Geometry: see drawing. Coordinates: mm, zero at the bounding-box minimum. A direction names the side the tool comes from. Give positions to 0.01 mm unless a question says otherwise; leave off trailing zeros. Loops run counter-clockwise (first coordinate to the right, second up) from the corner with the lowest first, then second, coordinate; pieces in that order, holes last. Notation, with made-up numbers: (-17.75, -3) - (-8.75, -3) arc R21 ccw to (-8.75, 36) - close; hole circle Ø7 at (-19.5, 39). An arc over 180 degrees is marked (long way). Use CSV: the item, a comma, the result in double quotes. Start each with the question number.
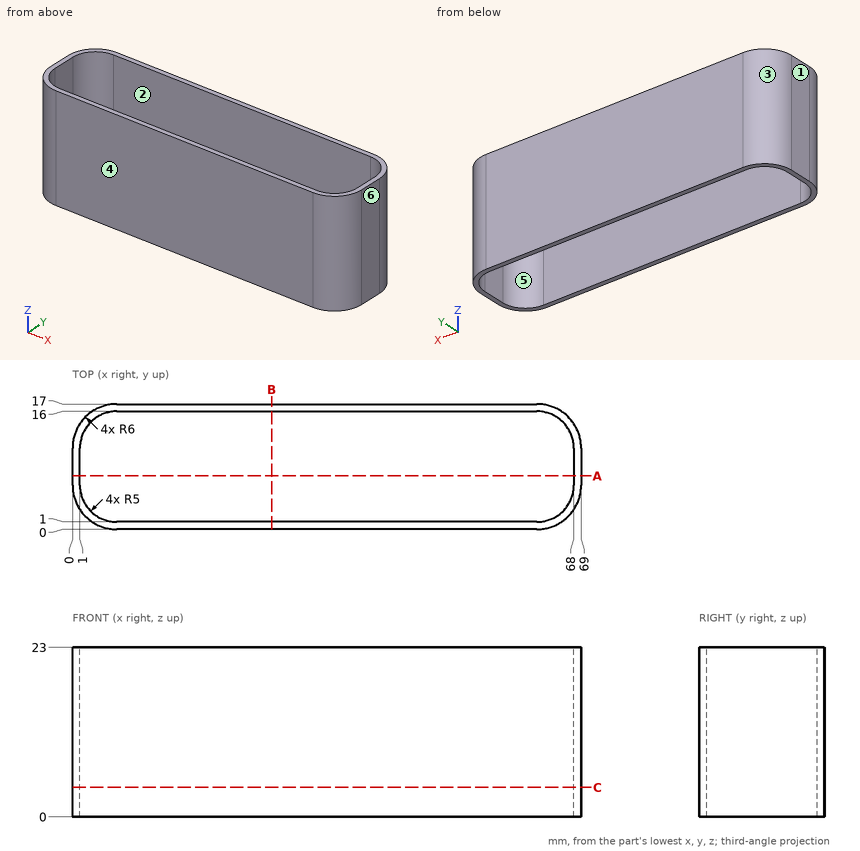
Item 1: Section C-C (z = 4). Output: boundary loops of the cut face in (x, y), plus the area to 3 significant figures.
Item 2: Section B-B (x = 27). Output: boundary loops of the cut face in (y, z).
Item 3: Pin query (flat end, axial travel): pin 1 Ø8 at (x, y) = (34, 11.5) entering from +Z. Return the tip coordinate at first contact, or that it passes through.
Item 4: Reachability of the marked faces 1 and 2 from +Z, -Z, +X, -X, +Y, -Y: full face, straight path, thin tool, end or side. Return the list, or none.
Item 5: Mould query, pull axis Y, two halves, no side actions, for the marked faces 3, 4, 5 and 6. Classes: pulls with the +Y half, pulls with the -Y half, needs draft (parallel to the pull), parting line crosses it, or undercut.
Item 6: Section A-A (y = 7.25). Output: boundary loops of the cut face in (x, z), plus the area to 3 significant figures.
Item 7: Ray query, probe 1 along Y at (x, z) = (15.5, 12.25); probe 2 along X at (y, z) = (7, 11); probe 3 along X at (y, z) = (13.75, 1.75). Return the intervals inside material, ascending.
Outcome:
1,outline,"(0, 6) arc R6 ccw to (6, 0) - (63, 0) arc R6 ccw to (69, 6) - (69, 11) arc R6 ccw to (63, 17) - (6, 17) arc R6 ccw to (0, 11) - close; hole (1, 6) arc R5 ccw to (6, 1) - (63, 1) arc R5 ccw to (68, 6) - (68, 11) arc R5 ccw to (63, 16) - (6, 16) arc R5 ccw to (1, 11) - close"
1,area,"159 mm2"
2,outline,"(0, 0) - (1, 0) - (1, 23) - (0, 23) - close; (16, 0) - (17, 0) - (17, 23) - (16, 23) - close"
3,pin 1,"passes through"
4,face 1,"+Z, -Z, -X, +Y, -Y"
4,face 2,"+Z, -Z"
5,face 3,"pulls with the +Y half"
5,face 4,"pulls with the -Y half"
5,face 5,"undercut"
5,face 6,"needs draft"
6,outline,"(0, 0) - (1, 0) - (1, 23) - (0, 23) - close; (68, 0) - (69, 0) - (69, 23) - (68, 23) - close"
6,area,"46.0 mm2"
7,probe 1,"y = 0 to 1, 16 to 17"
7,probe 2,"x = 0 to 1, 68 to 69"
7,probe 3,"x = 0.67 to 1.82, 67.18 to 68.33"
